from build123d import *

# Parameters (mm, degrees)
F0_R     = 3.8
F0_R_2   = 4.6
F1_DEPTH = 0.5


# Not quite as in the source:
# - a feature names something its author has since deleted; it is built from what else it names


with BuildPart() as f1:
    # F0 (on Top) → F1 (new body)
    with BuildSketch(Plane.XY):
        with BuildLine():
            ThreePointArc((24.3621806055, 39.2965673213), (24.8508286843, 41.6682755665), (26.2371806055, 43.6536735858))
            ThreePointArc((26.2371806055, 43.6536735858), (19.3621806055, 60.91551736), (12.4871806055, 43.6536735858))
            ThreePointArc((12.4871806055, 43.6536735858), (13.8735325268, 41.6682755665), (14.3621806055, 39.2965673213))
            Line((14.3621806055, 39.2965673213), (14.3621806055, -34.8549244096))
            ThreePointArc((14.3621806055, -34.8549244096), (14.1166056215, -37.9794551404), (13.3859113767, -41.0272552129))
            Line((13.3859113767, -41.0272552129), (-4.4496847801, -95.9983172384))
            ThreePointArc((-4.4496847801, -95.9983172384), (8.4471568034, -108.4941551178), (10.428313753, -90.646199933))
            ThreePointArc((10.428313753, -90.646199933), (8.0021901548, -87.6142160275), (7.9408744101, -83.7315310678))
            Line((7.9408744101, -83.7315310678), (13.6550613742, -66.1198446814))
            ThreePointArc((13.6550613742, -66.1198446814), (19.3621806055, -61.9715439224), (25.0692998369, -66.1198446814))
            Line((25.0692998369, -66.1198446814), (30.783486801, -83.7315310678))
            ThreePointArc((30.783486801, -83.7315310678), (30.7221710563, -87.6142160275), (28.2960474581, -90.646199933))
            ThreePointArc((28.2960474581, -90.646199933), (30.2772044076, -108.4941551178), (43.1740459911, -95.9983172384))
            Line((43.1740459911, -95.9983172384), (25.3384498343, -41.0272552129))
            ThreePointArc((25.3384498343, -41.0272552129), (24.6077555896, -37.9794551404), (24.3621806055, -34.8549244096))
            Line((24.3621806055, -34.8549244096), (24.3621806055, 39.2965673213))
        make_face()
        with Locations((5.0621806055, -99.08448264)):
            Circle(F0_R, mode=Mode.SUBTRACT)
        with Locations((33.6621806055, -99.08448264)):
            Circle(F0_R, mode=Mode.SUBTRACT)
        with Locations((19.3621806055, 50.91551736)):
            Circle(F0_R_2, mode=Mode.SUBTRACT)
    extrude(amount=F1_DEPTH)


solid = f1.part
The listing builds one solid part. Answer for the finished solid, in the listing's coordinates (mm). A direction names the side the tool comes from. Give positions to 0.01 mm unless a question says otherwise; leave off trailing zeros. Write each loop counter-clockwise with the first axis right and the second up, starting at its lowest first coordinate (ties: lowest second). Pieces come first, ordered by that corner, then holes. Notation, with made-up numbers: (10.5, 27) - (18.5, 27) arc R8 ccw to (18.5, 32) - close; hole circle Ø5 at (14.25, -16). An arc over 180 degrees is marked (long way). One line per question, with ' | ' between items. Start each with the question number.
1. For faces 1 (the face through (21, -43, 0)), 2 (the face through (10.758, -75.049, 0.246)), 3 (the face through (4.6, -68.1, 0.2)), determine the directions among +Z, -Z, +X, -X, +Y, -Y from which every point of the face is accessible in a straight line to the end or side of a thin tool.
2. Section D-D, the plane y = -51 is taken. Determine the outline of the cut face in (x, z), then the cut area to 3 significant figures.
3. Straight lines are drawn through the part: line 1 (X direction, y = -98.5, z = 0.35); line 2 (X direction, y = -41, z = 0.45); line 3 (X direction, y = -26.5, z = 0.4). For each, find the intervals that lie inside material, in ascending order.
4. Section A-A, the plane x = 16.5 is taken. Determine the outline of the cut face in (y, z), then the cut area to 3 significant figures.
5. Section B-B, the plane z = 0.4 is taken. Determine the outline of the cut face in (x, y), then the cut area to 3 significant figures.
6. Given P1, Ø4.5, axis at x = 5.06, y = -99.08, coming from the -Z side, flat-ended and moving along its own axis, determine where the tip first touches the part or whether it passes through.
7. Section C-C, the plane y = 29.5 is taken. Determine the outline of the cut face in (x, z).
8. Determine the mould class of faces 4 (the face through (21, -43, 0.5)), 5 (the face through (34.38, -68.9, 0.25)) for opening direction Y: +Y half, -Y half, draft (parallel to the pull), parting line (faces both ways), or undercut.
Result:
1) face 1: -Z, +X, -X, +Y, -Y | face 2: +Z, -Z | face 3: +Z, -Z, -X
2) outline: (10.15, 0) - (28.57, 0) - (28.57, 0.5) - (10.15, 0.5) - close | area: 9.21 mm2
3) line 1: x = -4.92 to 1.31, 8.82 to 15.05, 23.68 to 29.91, 37.42 to 43.65 | line 2: x = 13.39 to 25.33 | line 3: x = 14.36 to 24.36
4) outline: (-62.7, 0) - (47.31, 0) - (47.31, 0.5) - (-62.7, 0.5) - close; (54.52, 0) - (60.5, 0) - (60.5, 0.5) - (54.52, 0.5) - close | area: 58.0 mm2
5) outline: (-4.45, -96) arc R10 ccw (long way) to (10.43, -90.65) arc R6 cw to (7.94, -83.73) - (13.66, -66.12) arc R6 cw to (25.07, -66.12) - (30.78, -83.73) arc R6 cw to (28.3, -90.65) arc R10 ccw (long way) to (43.17, -96) - (25.34, -41.03) arc R20 cw to (24.36, -34.85) - (24.36, 39.3) arc R6 cw to (26.24, 43.65) arc R10 ccw (long way) to (12.49, 43.65) arc R6 cw to (14.36, 39.3) - (14.36, -34.85) arc R20 cw to (13.39, -41.03) - close; hole circle Ø7.6 at (5.06, -99.08); hole circle Ø9.2 at (19.36, 50.92); hole circle Ø7.6 at (33.66, -99.08) | area: 2,500 mm2
6) P1: passes through
7) outline: (14.36, 0) - (24.36, 0) - (24.36, 0.5) - (14.36, 0.5) - close
8) face 4: draft | face 5: undercut
